Source: CAD feature listing. Evaluate the final solid. Frame: model axes, mm. Face numbers are marked on the shaded views. Round coordinates to 2 decimals unless told otherwise and drop trailing zeros. Loops run counter-clockwise (first coordinate to the right, second up) from the corner with the lowest first, then second, coordinate; pieces in that order, holes last. Notation, with made-up numbers: (16.5, 35.25) -> (32.5, 35.25) arc R24 ccw to (32.5, 61.25) -> close; hole circle Ø3 at (26.5, -34). An arc over 180 degrees is marked (long way). Write item = value, one per line.
from build123d import *

# Parameters (mm, degrees)
F0_W           = 127
F0_H           = 50.8
F1_DEPTH       = 76.2
F3_D           = 12.7
F3_DEPTH       = 12.7
F3_CSINK_D     = 19.05
F3_CSINK_ANGLE = 82
F3_TIP         = 3.8154649308
F4_D           = 12.7
F4_CSINK_D     = 25.4
F4_CSINK_ANGLE = 82
F5_D           = 12.7
F6_D           = 6.35
F6_DEPTH       = 6.35
F6_CSINK_D     = 9.525
F6_CSINK_ANGLE = 82
F6_TIP         = 1.9077324654


with BuildPart() as f1:
    # F0 (on Front) → F1 (new body)
    with BuildSketch(Plane.XZ):
        with Locations((-63.5, 25.4)):
            Rectangle(F0_W, F0_H)
    extrude(amount=F1_DEPTH)

    # F3
    with Locations(Plane.XZ.offset(76.2)):
        with Locations((-107.95, 25.4)):
            CounterSinkHole(F3_D / 2, F3_CSINK_D / 2, depth=F3_DEPTH, counter_sink_angle=F3_CSINK_ANGLE)
            with Locations((0, 0, -(F3_DEPTH + F3_TIP / 2))):  # 118° drill point
                Cone(0, F3_D / 2, F3_TIP, mode=Mode.SUBTRACT)

    # F4 (through all)
    with Locations(Plane.XZ.offset(76.2)):
        with Locations((-82.55, 25.4)):
            CounterSinkHole(F4_D / 2, F4_CSINK_D / 2, counter_sink_angle=F4_CSINK_ANGLE)

    # F5 (through all)
    with Locations(Plane.XZ.offset(76.2)):
        with Locations((-50.8, 25.4)):
            Hole(F5_D / 2)

    # F6
    with Locations(Plane.XZ.offset(76.2)):
        with Locations((-19.05, 25.4)):
            CounterSinkHole(F6_D / 2, F6_CSINK_D / 2, depth=F6_DEPTH, counter_sink_angle=F6_CSINK_ANGLE)
            with Locations((0, 0, -(F6_DEPTH + F6_TIP / 2))):  # 118° drill point
                Cone(0, F6_D / 2, F6_TIP, mode=Mode.SUBTRACT)


solid = f1.part
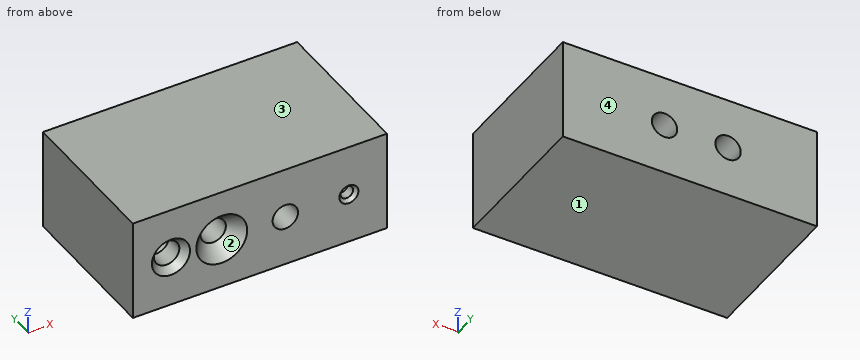
1. Section query B-B (x = -46). Return the cut outline in (y, z).
Evaluation:
outline = (-76.2, 0) -> (0, 0) -> (0, 21.24) -> (-76.2, 21.24) -> close; (-76.2, 29.56) -> (0, 29.56) -> (0, 50.8) -> (-76.2, 50.8) -> close
2. Mould query, pull axis Z, two halves, no side actions, for the marked faces 1, 2, 3 and 4. Classes: released by +Z, released by -Z, zero draft, split by the parting line, or undercut.
Evaluation:
face_1 = released by -Z
face_2 = undercut
face_3 = released by +Z
face_4 = zero draft
3. Contact query for a flat-ended pin moving along its axis: pin 1 Ø7.5 at (x, z) = (-19.05, 25.4) entering from -Y. Output: stop coordinate, or through.
Evaluation:
pin_1 = -75.04
4. Section query A-A (x = -82.55). Return the cut outline in (y, z), then the cut area to 3 significant figures.
Evaluation:
outline = (-76.2, 0) -> (0, 0) -> (0, 19.05) -> (-68.9, 19.05) -> (-76.2, 12.7) -> close; (-76.2, 38.1) -> (-68.9, 31.75) -> (0, 31.75) -> (0, 50.8) -> (-76.2, 50.8) -> close
area = 2,860 mm²
5. Line query: probe 1 along Z at (x, y) = (-50.8, -57); probe 2 along X at (y, z) = (-68, 22.5); probe 3 along Z at (x, y) = (-55, -52.5). Output: solid intervals per line, ascending. Write a range as from..to.
Evaluation:
probe_1 = 0..19.05, 31.75..50.8
probe_2 = -127..-113.6, -102.3..-88.2, -76.9..-56.45, -45.15..0
probe_3 = 0..20.64, 30.16..50.8
